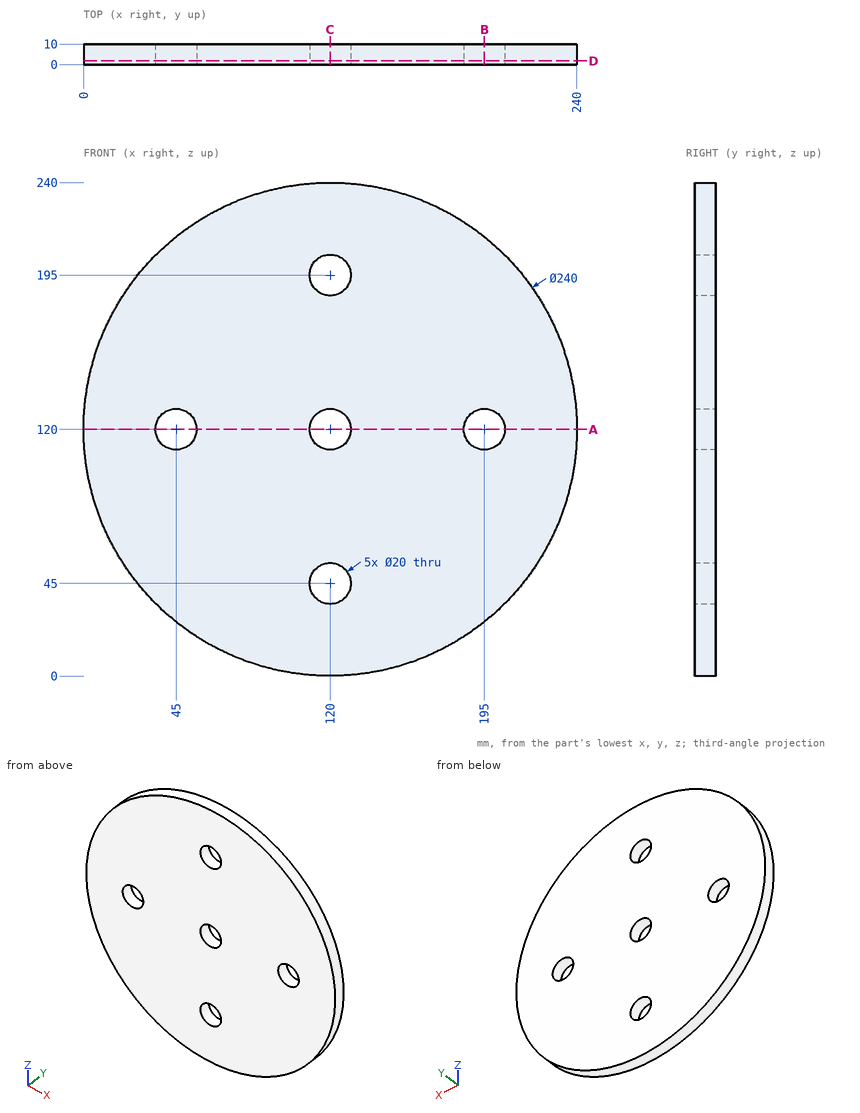
Study the drawing (mm; zero at the part's minimum x, y, z) and answer. Give positions to 0.01 mm unless a question says otherwise; leave off trailing zeros. Loops run counter-clockwise (first coordinate to the right, second up) from the corner with the lowest first, then second, coordinate; pieces in that order, holes last. Notation, with made-up numbers: M -19,45.5 L -15,45.5 A23 cw -15,54.5 Z; hole C 13,42 d4. An arc over 180 degrees is marked long. Answer as CSV lines item,"result".
Item 1: The part is cut by section D-D (y = 1.75). Give the vertices of the cut face in (x, z).
Values follow:
outline,"C 120,120 d240; hole C 45,120 d20; hole C 120,45 d20; hole C 120,120 d20; hole C 120,195 d20; hole C 195,120 d20"
Item 2: The part is cut by section C-C (x = 120). Give the vertices of the cut face in (y, z).
Values follow:
outline,"M 0,0 L 10,0 L 10,35 L 0,35 Z; M 0,55 L 10,55 L 10,110 L 0,110 Z; M 0,130 L 10,130 L 10,185 L 0,185 Z; M 0,205 L 10,205 L 10,240 L 0,240 Z"
Item 3: The part is cut by section B-B (x = 195). Give the vertices of the cut face in (y, z), and give its area (3 significant figures).
Values follow:
outline,"M 0,26.33 L 10,26.33 L 10,110 L 0,110 Z; M 0,130 L 10,130 L 10,213.67 L 0,213.67 Z"
area,"1,670 mm^2"
Item 4: Given pin 1 Ø2 at (x, y) = (94.5, 7) entering from +Z; pin 2 Ø16 at (x, z) = (120, 45) entering from +Y; pin 3 Ø6 at (x, y) = (138.5, 7) entering from -Z; pin 4 Ø5 at (y, z) = (5.5, 202) entering from +X, each flat-ended and moving along its own axis, determine where each tip first touches the part or whether it passes through.
Values follow:
pin 1,"stops at z = 237.47"
pin 2,"passes through"
pin 3,"stops at z = 1.01"
pin 4,"stops at x = 209.89"
Item 5: The part is cut by section A-A (z = 120). Give the vertices of the cut face in (x, y).
Values follow:
outline,"M 0,0 L 35,0 L 35,10 L 0,10 Z; M 55,0 L 110,0 L 110,10 L 55,10 Z; M 130,0 L 185,0 L 185,10 L 130,10 Z; M 205,0 L 240,0 L 240,10 L 205,10 Z"
Item 6: Straight lines are drawn through the part: line 1 along X through (y, z) = (3.75, 120); line 2 along X through (y, z) = (8.25, 124); line 3 along Z through (x, y) = (118.5, 5.5). For each, find the intervals that lie inside material, in ascending order. Write a range as [from, to].
Values follow:
line 1,"x = [0, 35], [55, 110], [130, 185], [205, 240]"
line 2,"x = [0.07, 35.83], [54.17, 110.83], [129.17, 185.83], [204.17, 239.93]"
line 3,"z = [0.01, 35.11], [54.89, 110.11], [129.89, 185.11], [204.89, 239.99]"
